For this review, take the finished solid that the model builds, in its own axes (mm). A direction names the side the tool comes from. Coordinates: 2 decimals unless noted, no trailing zeros. Loops run counter-clockwise (first coordinate to the right, second up) from the corner with the lowest first, then second, coordinate; pieces in that order, holes last.
1. To check wall thickness, follow probe 1 along Y at (x, z) = (0, 4); probe 2 along Y at (x, z) = (0, 14); probe 3 along X at (y, z) = (0, 26.25). State the ranges of each line that lie inside material, in increasing order.
2. Take a section at C-C, the plane x = 23. State the section outline as (y, z) points, then the cut area to 3 significant figures.
3. Clearance check with flat-ended pins moving along their axes: P1, Ø1.5, axis at y = 25, z = 7, coming from the +X side; P2, Ø6, axis at y = 5.5, z = 14.5, coming from the -X side; P3, Ø6, axis at x = -8.5, z = 20, coming from the +Y side. State where each tip first meets the part, or that it passes through.
4. Take a section at D-D, the plane z = 16.5. State the section outline as (x, y) points, then the cut area to 3 significant figures.
5. Mouldability with a two-part tool opening along X and no side actions: class faces 3 (the face through (-1.42, -3.92, 20)), 4 (the face through (1, 7, 0)), 5 (the face through (-28, -21, 5)) as pulls with the +X half, pulls with the -X half, needs draft (parallel to the pull), parting line crosses it, or undercut.
6. Take a section at A-A, the plane y = 0. State the section outline as (x, z) points, then the cut area to 4 significant figures.
7. Machinability: for faces 1 (the face through (-4, 5, 35)), 2 (the face through (-6, 0, 27)), which of the approach directions +Z, -Z, +X, -X, +Y, -Y give a long, thin tool a straight path to every point of the face, cutting with its end or side? Answer none if there is none.
```python
from build123d import *

# Parameters (mm, degrees)
SKETCH1_R           = 35
SKETCH1_R_2         = 6
SKETCH1_R_3         = 2.75
BOSS_EXTRUDE1_DEPTH = 10
SKETCH2_R           = 22
SKETCH2_R_2         = 6
BOSS_EXTRUDE2_DEPTH = 35
SKETCH3_R           = 12
SKETCH3_R_2         = 4
BOSS_EXTRUDE3_DEPTH = 20


with BuildPart() as part:
    # Sketch1 → Boss-Extrude1 (new body)
    with BuildSketch(Plane.XY):
        Circle(SKETCH1_R)
        Circle(SKETCH1_R_2, mode=Mode.SUBTRACT)
        with Locations((22.5, 0)):
            Circle(SKETCH1_R_3, mode=Mode.SUBTRACT)
        with Locations((0, 22.5)):
            Circle(SKETCH1_R_3, mode=Mode.SUBTRACT)
        with Locations((-22.5, 0)):
            Circle(SKETCH1_R_3, mode=Mode.SUBTRACT)
        with Locations((0, -22.5)):
            Circle(SKETCH1_R_3, mode=Mode.SUBTRACT)
    extrude(amount=BOSS_EXTRUDE1_DEPTH)

    # Sketch2 → Boss-Extrude2 (add)
    with BuildSketch(Plane.XY):
        with Locations(Location((0, 0, 0), (0, 0, 173.031799207))):
            Circle(SKETCH2_R)
        Circle(SKETCH2_R_2, mode=Mode.SUBTRACT)
    extrude(amount=BOSS_EXTRUDE2_DEPTH)

    # Sketch3 → Boss-Extrude3 (add)
    with BuildSketch(Plane.XY):
        Circle(SKETCH3_R)
        Circle(SKETCH3_R_2, mode=Mode.SUBTRACT)
    extrude(amount=BOSS_EXTRUDE3_DEPTH)


solid = part.part
```
Results list:
1. probe 1: y = -35 to -25.25, -22 to -4, 4 to 22, 25.25 to 35
1. probe 2: y = -22 to -4, 4 to 22
1. probe 3: x = -22 to -6, 6 to 22
2. outline: (-26.38, 0) - (-2.7, 0) - (-2.7, 10) - (-26.38, 10) - close; (2.7, 0) - (26.38, 0) - (26.38, 10) - (2.7, 10) - close
2. area: 474 mm2
3. P1: stops at x = 25.24
3. P2: stops at x = -21.86
3. P3: stops at y = 21.3
4. outline: circle Ø44 at (0, 0); hole circle Ø8 at (0, 0)
4. area: 1,470 mm2
5. face 3: undercut
5. face 4: needs draft
5. face 5: parting line crosses it
6. outline: (-35, 0) - (-25.25, 0) - (-25.25, 10) - (-35, 10) - close; (-22, 0) - (-4, 0) - (-4, 20) - (-6, 20) - (-6, 35) - (-22, 35) - close; (4, 0) - (22, 0) - (22, 35) - (6, 35) - (6, 20) - (4, 20) - close; (25.25, 0) - (35, 0) - (35, 10) - (25.25, 10) - close
6. area: 1,395 mm2
7. face 1: +Z, +X, -X, +Y, -Y
7. face 2: +Z
